Source: three-view drawing plus pictorial views. Frame: mm from the lowest corner of the part. A direction names the side the tool comes from. Coordinates: 2 decimals unless noted, no trailing zeros. Order: outer loops, then holes, each group sorted by start corner. A loop starts at its lowest first (then second) coordinate and runs counter-clockwise, first axis right, second up. Notation, with made-up numbers: M 64.25,89.25 L 111.25,89.25 A34 ccw 111.25,124.25 Z; hole C 53.25,1 d10. An arc over 180 degrees is marked long. Use CSV: the item, a comma, the result in double quotes. Start each with the question number.
Q1. Section query C-C, the plane z = 22.5. Output: boundary loops of the cut face in (x, y), and give its area (3 significant figures).
Q2. Section query B-B, the plane y = 35. Output: boundary loops of the cut face in (x, z).
Q3. First-contact query: P1, Ø3, axis at y = 18, z = 21.5, coming from the +X side; P2, Ø5, axis at x = 14, z = 34, coming from the +Y side. Flat tips, straight axial feed; report the tip coordinate or a pass-through.
Q4. Access query for the marked faces 1 and 2. Directions: +Z, -Z, +X, -X, +Y, -Y. A direction counts if a zero-diameter tool reaches every point of the face in a straight line with its end or side. Return the directions, or none.
Q5. Section query D-D, the plane y = 48. Output: boundary loops of the cut face in (x, z).
Q6. Ray query, probe 1 along Y at (x, z) = (2.9, 20); probe 2 along Y at (x, z) = (9, 28.5). Return the intervals inside material, ascending.
Q7. Section query A-A, the plane x = 14. Output: boundary loops of the cut face in (y, z).
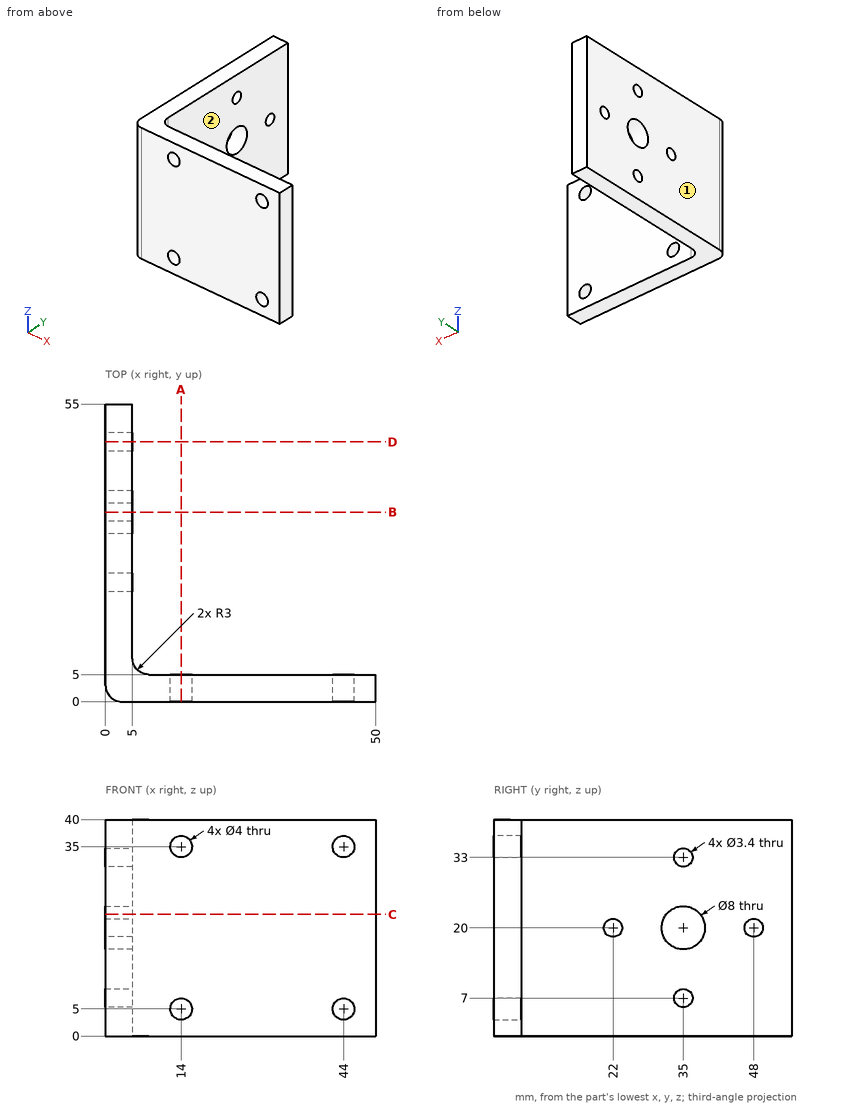
Responses:
1,outline,"M 0,3 A3 ccw 3,0 L 50,0 L 50,5 L 8,5 A3 cw 5,8 L 5,31.88 L 0,31.88 Z; M 0,38.12 L 5,38.12 L 5,55 L 0,55 Z"
1,area,"469 mm²"
2,outline,"M 0,0 L 5,0 L 5,5.3 L 0,5.3 Z; M 0,8.7 L 5,8.7 L 5,16 L 0,16 Z; M 0,24 L 5,24 L 5,31.3 L 0,31.3 Z; M 0,34.7 L 5,34.7 L 5,40 L 0,40 Z"
3,P1,"stops at x = 5"
3,P2,"stops at y = 5"
4,face 1,"+Z, -Z, -X, +Y, -Y"
4,face 2,"+Z, -Z, +X, +Y"
5,outline,"M 0,0 L 5,0 L 5,18.3 L 0,18.3 Z; M 0,21.7 L 5,21.7 L 5,40 L 0,40 Z"
6,probe 1,"y = 0 to 20.3, 23.7 to 31, 39 to 46.3, 49.7 to 55"
6,probe 2,"y = 0 to 5"
7,outline,"M 0,0 L 5,0 L 5,3 L 0,3 Z; M 0,7 L 5,7 L 5,33 L 0,33 Z; M 0,37 L 5,37 L 5,40 L 0,40 Z"
